Verification items for the finished model (mm, model axes). A direction names the side the tool comes from. Coordinates: 2 decimals unless noted, no trailing zeros. Write each loop counter-clockwise with the first axis right and the second up, starting at its lowest first coordinate (ties: lowest second). Pieces come first, ordered by that corner, then holes. Notation, with made-up numbers: (25.25, 56) -> (40.25, 56) arc R25 ccw to (40.25, 84) -> close; hole circle Ø5 at (-34.5, 79). An arc over 180 degrees is marked (long way). Answer in a Markdown table with one row per item.
```python
from build123d import *

# Parameters (mm, degrees)
F0_R           = 55
F0_R_2         = 3
F1_DEPTH       = 50
F2_R           = 38.5
F2_R_2         = 3
F3_DEPTH       = 33
F5_D           = 6.6
F5_CBORE_D     = 11.25
F5_CBORE_DEPTH = 6


with BuildPart() as f1:
    # F0 (on Top) → F1 (new body)
    with BuildSketch(Plane.XY):
        Circle(F0_R)
        with BuildLine():
            ThreePointArc((28.0281341694, -14.45), (25.8045913047, -17.3477774789), (22.430057958, -15.95))
            Line((22.430057958, -15.95), (2.5980762114, -27.4))
            ThreePointArc((2.5980762114, -27.4), (2.8977774789, -28.1235428647), (3, -28.9))
            ThreePointArc((3, -28.9), (-0.7764571353, -31.7977774789), (-2.5980762114, -27.4))
            Line((-2.5980762114, -27.4), (-22.430057958, -15.95))
            ThreePointArc((-22.430057958, -15.95), (-27.6262103807, -15.95), (-25.0281341694, -11.45))
            Line((-25.0281341694, -11.45), (-25.0281341694, 11.45))
            ThreePointArc((-25.0281341694, 11.45), (-27.6262103807, 15.95), (-22.430057958, 15.95))
            Line((-22.430057958, 15.95), (-2.5980762114, 27.4))
            ThreePointArc((-2.5980762114, 27.4), (-0.7764571353, 31.7977774789), (3, 28.9))
            ThreePointArc((3, 28.9), (2.8977774789, 28.1235428647), (2.5980762114, 27.4))
            Line((2.5980762114, 27.4), (22.430057958, 15.95))
            ThreePointArc((22.430057958, 15.95), (25.8045913047, 17.3477774789), (28.0281341694, 14.45))
            ThreePointArc((28.0281341694, 14.45), (27.1494545129, 12.3286796564), (25.0281341694, 11.45))
            Line((25.0281341694, 11.45), (25.0281341694, -11.45))
            ThreePointArc((25.0281341694, -11.45), (27.1494545129, -12.3286796564), (28.0281341694, -14.45))
        make_face(mode=Mode.SUBTRACT)
        with BuildLine():
            Line((2.5980762114, -27.4), (22.430057958, -15.95))
            ThreePointArc((22.430057958, -15.95), (22.430057958, -12.95), (25.0281341694, -11.45))
            Line((25.0281341694, -11.45), (25.0281341694, 11.45))
            ThreePointArc((25.0281341694, 11.45), (22.430057958, 12.95), (22.430057958, 15.95))
            Line((22.430057958, 15.95), (2.5980762114, 27.4))
            ThreePointArc((2.5980762114, 27.4), (0, 25.9), (-2.5980762114, 27.4))
            Line((-2.5980762114, 27.4), (-22.430057958, 15.95))
            ThreePointArc((-22.430057958, 15.95), (-22.1303566905, 15.2264571353), (-22.0281341694, 14.45))
            ThreePointArc((-22.0281341694, 14.45), (-22.9068138258, 12.3286796564), (-25.0281341694, 11.45))
            Line((-25.0281341694, 11.45), (-25.0281341694, -11.45))
            ThreePointArc((-25.0281341694, -11.45), (-22.9068138258, -12.3286796564), (-22.0281341694, -14.45))
            ThreePointArc((-22.0281341694, -14.45), (-22.1303566905, -15.2264571353), (-22.430057958, -15.95))
            Line((-22.430057958, -15.95), (-2.5980762114, -27.4))
            ThreePointArc((-2.5980762114, -27.4), (0, -25.9), (2.5980762114, -27.4))
        make_face()
        Circle(F0_R_2, mode=Mode.SUBTRACT)
    extrude(amount=F1_DEPTH)

    # F2 (on face) → F3 (cut)
    with BuildSketch(Plane.XY.offset(50)):
        Circle(F2_R)
        with Locations((-25.0281341694, -14.45)):
            Circle(F2_R_2, mode=Mode.SUBTRACT)
        with Locations((0, -28.9)):
            Circle(F2_R_2, mode=Mode.SUBTRACT)
        with Locations((25.0281341694, -14.45)):
            Circle(F2_R_2, mode=Mode.SUBTRACT)
        with Locations((-25.0281341694, 14.45)):
            Circle(F2_R_2, mode=Mode.SUBTRACT)
        Circle(F2_R_2, mode=Mode.SUBTRACT)
        with Locations((25.0281341694, 14.45)):
            Circle(F2_R_2, mode=Mode.SUBTRACT)
        with Locations((0, 28.9)):
            Circle(F2_R_2, mode=Mode.SUBTRACT)
    extrude(amount=-F3_DEPTH, mode=Mode.SUBTRACT)

    # F5 (through all)
    with Locations(Plane.XY.offset(17)):
        with Locations((-25.0281341694, 14.45), (-25.0281341694, -14.45), (0, -28.9), (25.0281341694, -14.45), (25.0281341694, 14.45), (0, 28.9), (0, 0)):
            CounterBoreHole(F5_D / 2, F5_CBORE_D / 2, F5_CBORE_DEPTH)


solid = f1.part
```
1. Section check A-A, the plane x = 0. State how many separate pieces and enclosed holes the cut face has, plus the area to 3 significant figures.
Geometry says:
| item | result |
|---|---|
| separate pieces | 4 |
| enclosed holes | 0 |
| area | 2,540 mm^2 |
2. Depth check by flat-ended pin: P1, Ø7.5, axis at x = 25.03, y = -14.45, coming from the +Z side; P2, Ø8, axis at y = -6, z = 32.5, coming from the -X side; P3, Ø9, axis at x = 2.5, y = -29.5, coming from the +Z side; P4, Ø5.5, axis at x = 0, y = 28.9, coming from the -Z side. Enter the tip coordinate at first touch or a pass-through.
Geometry says:
| item | result |
|---|---|
| P1 | z = 11 |
| P2 | x = -54.96 |
| P3 | z = 17 |
| P4 | through |
3. Tool access check on faces 1 (the cylindrical face through (30.224, -16.604, 14.042)), 2 (the cylindrical face through (0.72, 25.68, 5.42)). Record the directions out of +Z, -Z, +X, -X, +Y, -Y that give a thin tool (end or side, any length) a straight path to the whole face; none if there is none.
Geometry says:
| item | result |
|---|---|
| face 1 | +Z |
| face 2 | +Z, -Z |
4. Section check D-D, the plane x = 27. Record the boundary of the cut face in (y, z), plus the area to 3 significant figures.
Geometry says:
| item | result |
|---|---|
| outline | (-47.92, 0) -> (-17.1, 0) -> (-17.1, 11) -> (-19.72, 11) -> (-19.72, 17) -> (-27.45, 17) -> (-27.45, 50) -> (-47.92, 50) -> close; (-11.8, 0) -> (11.8, 0) -> (11.8, 11) -> (9.18, 11) -> (9.18, 17) -> (-9.18, 17) -> (-9.18, 11) -> (-11.8, 11) -> close; (17.1, 0) -> (47.92, 0) -> (47.92, 50) -> (27.45, 50) -> (27.45, 17) -> (19.72, 17) -> (19.72, 11) -> (17.1, 11) -> close |
| area | 2,740 mm^2 |
5. Section check C-C, the plane y = 14.45. Record the boundary of the cut face in (x, z).
Geometry says:
| item | result |
|---|---|
| outline | (-53.07, 0) -> (-28.33, 0) -> (-28.33, 11) -> (-30.65, 11) -> (-30.65, 17) -> (-35.69, 17) -> (-35.69, 50) -> (-53.07, 50) -> close; (-21.73, 0) -> (21.73, 0) -> (21.73, 11) -> (19.4, 11) -> (19.4, 17) -> (-19.4, 17) -> (-19.4, 11) -> (-21.73, 11) -> close; (28.33, 0) -> (53.07, 0) -> (53.07, 50) -> (35.69, 50) -> (35.69, 17) -> (30.65, 17) -> (30.65, 11) -> (28.33, 11) -> close |
6. Thickness scan on line 1 (Y direction, x = 0, z = 13) (3 decimals); line 2 (Y direction, x = 0, z = 6.5); line 3 (X direction, y = -14, z = 14). Record the ranges inside material, lowest first. Write a range as from..to.
Geometry says:
| item | result |
|---|---|
| line 1 | -55..-34.525, -23.275..-5.625, 5.625..23.275, 34.525..55 |
| line 2 | -55..-32.2, -25.6..-3.3, 3.3..25.6, 32.2..55 |
| line 3 | -53.19..-30.64, -19.42..19.42, 30.64..53.19 |
7. Section check B-B, the plane y = 0. Record the boundary of the cut face in (x, z) (3 decimals).
Geometry says:
| item | result |
|---|---|
| outline | (-55, 0) -> (-3.3, 0) -> (-3.3, 11) -> (-5.625, 11) -> (-5.625, 17) -> (-38.5, 17) -> (-38.5, 50) -> (-55, 50) -> close; (3.3, 0) -> (55, 0) -> (55, 50) -> (38.5, 50) -> (38.5, 17) -> (5.625, 17) -> (5.625, 11) -> (3.3, 11) -> close |
